Source: CAD feature listing. Evaluate the final solid. Frame: model axes, mm. A direction names the side the tool comes from. Coordinates: 2 decimals unless noted, no trailing zeros. Loops run counter-clockwise (first coordinate to the right, second up) from the corner with the lowest first, then second, coordinate; pieces in that order, holes last.
Item 1: Line query: probe 1 along Z at (x, y) = (0, -4); probe 2 along Z at (x, y) = (29.5, 5); probe 3 along Z at (x, y) = (20, -7). Output: solid intervals per line, ascending.
Item 2: Section query D-D, the plane y = 16. Return the cut outline in (x, z).
Item 3: Pin query (flat end, axial travel): pin 1 Ø4 at (y, z) = (-14.5, 10.5) entering from -X; pin 2 Ø1 at (x, z) = (0.5, 16) entering from +Y; pin 3 Ø8 at (x, z) = (3.5, 5.5) entering from +Y. Return the tip coordinate at first contact, or that it passes through.
Item 4: Reachability of faces 1 (the flat face through (4, -8, 4)), 2 (the flat face through (-2, -12.99, 6)), 3 (the cylindrical face through (11.5, -22.2, 20.4)), 4 (the cylindrical face through (-0.434, -11.27, 2.548)) from +Z, -Z, +X, -X, +Y, -Y: full face, straight path, thin tool, end or side. Return the list, or none.
Item 5: Section query A-A, the plane x = 0. State how many separate pieces and enclosed holes the cut face has, then the cut area to 3 significant figures.
Item 6: Section query B-B, the plane z = 4.5. Return the cut outline in (x, y).
Item 7: Section query C-C, the plane y = 1. Return the cut outline in (x, z), then the cut area to 3 significant figures.
Item 8: Pull-direction query (X, two-part tool) for faces 5 (the flat face through (0, -8, 9)), 6 (the flat face through (11.198, -6.586, 4.93)), 7 (the flat face through (0, -14, 10)); classes: +X half, -X half, draft (parallel to the pull), parting line (faces both ways), or undercut.
```python
from build123d import *

# Parameters (mm, degrees)
SKETCH001_R     = 32.5
PAD001_DEPTH    = 3
SKETCH002_R     = 25
PAD002_DEPTH    = 15
SKETCH003_R     = 32.5
PAD003_DEPTH    = 3
PAD_DEPTH       = 10
POCKET_DEPTH    = 31
SKETCH005_W     = 8
SKETCH005_H     = 3.5
POCKET001_DEPTH = 9
SKETCH006_R     = 2
POCKET002_DEPTH = 7
SKETCH007_W     = 2.5
SKETCH007_H     = 5
POCKET003_DEPTH = 5
POCKET004_DEPTH = 13


with BuildPart() as obj1:
    # Sketch001 → Pad001 (new body)
    with BuildSketch(Plane.XY):
        Circle(SKETCH001_R)
    extrude(amount=PAD001_DEPTH)

    # Sketch002 (on Sketch) → Pad002 (join)
    with BuildSketch(Plane.XY.offset(3)):
        Circle(SKETCH002_R)
    extrude(amount=PAD002_DEPTH)

    # Sketch003 (on Face5 of Pad002) → Pad003 (join)
    with BuildSketch(Plane.XY.offset(18)):
        Circle(SKETCH003_R)
    extrude(amount=PAD003_DEPTH)


with BuildPart() as obj1_1:
    # Body placement: moved
    add(obj1.part.moved(Location((0, 0, 10))))


with BuildPart() as base:
    # Sketch → Pad (new body)
    with BuildSketch(Plane.XY):
        Polygon((15, 0), (7.5, 12.990381), (-7.5, 12.990381), (-15, 0), (-7.5, -12.990381), (7.5, -12.990381), align=None)
    extrude(amount=PAD_DEPTH)

    # Boolean: union obj1
    add(obj1_1.part)

    # Sketch004 (on Sketch) → Pocket (cut)
    with BuildSketch(Plane(origin=(0, 0, 0), x_dir=(1, 0, 0), z_dir=(0, 0, -1))):
        with BuildLine():
            ThreePointArc((-1.661325, 2), (0, -2.6), (1.661325, 2))
            Line((-1.661325, 2), (1.661325, 2))
        make_face()
    extrude(amount=-POCKET_DEPTH, mode=Mode.SUBTRACT)

    # Sketch005 (on Face8 of Pocket) → Pocket001 (cut)
    with BuildSketch(Plane(origin=(0, 0, 0), x_dir=(1, 0, 0), z_dir=(0, 0, -1))):
        with Locations((0, 7.75)):
            Rectangle(SKETCH005_W, SKETCH005_H)
    extrude(amount=-POCKET001_DEPTH, mode=Mode.SUBTRACT)

    # Sketch006 (on Face13 of Pocket001) → Pocket002 (cut)
    with BuildSketch(Plane.XZ.offset(12.990381)):
        with Locations((0, 4.5)):
            Circle(SKETCH006_R)
    extrude(amount=-POCKET002_DEPTH, mode=Mode.SUBTRACT)

    # Sketch007 (on Face22 of Pocket002) → Pocket003 (cut)
    with BuildSketch(Plane(origin=(0, 0, 9), x_dir=(1, 0, 0), z_dir=(0, 0, -1))):
        with Locations((3.25, -25)):
            Rectangle(SKETCH007_W, SKETCH007_H)
        with Locations((-3.25, -25)):
            Rectangle(SKETCH007_W, SKETCH007_H)
    extrude(amount=-POCKET003_DEPTH, mode=Mode.SUBTRACT)

    # Sketch006 (on Face13 of Pocket001) → Pocket004 (cut)
    with BuildSketch(Plane.XZ.offset(12.990381)):
        with Locations((0, 4.5)):
            Circle(SKETCH006_R)
    extrude(amount=-POCKET004_DEPTH, mode=Mode.SUBTRACT)


solid = base.part
```
Verdict:
1. probe 1: z = 0 to 2.5, 6.5 to 31
1. probe 2: z = 10 to 13, 28 to 31
1. probe 3: z = 10 to 31
2. outline: (-28.29, 10) - (28.29, 10) - (28.29, 13) - (19.21, 13) - (19.21, 28) - (28.29, 28) - (28.29, 31) - (-28.29, 31) - (-28.29, 28) - (-19.21, 28) - (-19.21, 13) - (-28.29, 13) - close
3. pin 1: stops at x = -30
3. pin 2: stops at y = 25
3. pin 3: stops at y = 12.99
4. face 1: -Z
4. face 2: -Z, +X, -X, -Y
4. face 3: none
4. face 4: -Y
5. separate pieces: 4
5. enclosed holes: 0
5. area: 1,200 mm2
6. outline: (-15, 0) - (-7.5, -12.99) - (-2, -12.99) - (-2, -9.5) - (-4, -9.5) - (-4, -6) - (-2, -6) - (-2, -1.66) arc R2.6 cw (long way) to (2, -1.66) - (2, -6) - (4, -6) - (4, -9.5) - (2, -9.5) - (2, -12.99) - (7.5, -12.99) - (15, 0) - (7.5, 12.99) - (-7.5, 12.99) - close
7. outline: (-32.48, 10) - (-14.42, 10) - (-14.42, 0) - (-2.4, 0) - (-2.4, 31) - (-32.48, 31) - (-32.48, 28) - (-24.98, 28) - (-24.98, 13) - (-32.48, 13) - close; (2.4, 0) - (14.42, 0) - (14.42, 10) - (32.48, 10) - (32.48, 13) - (24.98, 13) - (24.98, 28) - (32.48, 28) - (32.48, 31) - (2.4, 31) - close
7. area: 1,280 mm2
8. face 5: undercut
8. face 6: +X half
8. face 7: draft
